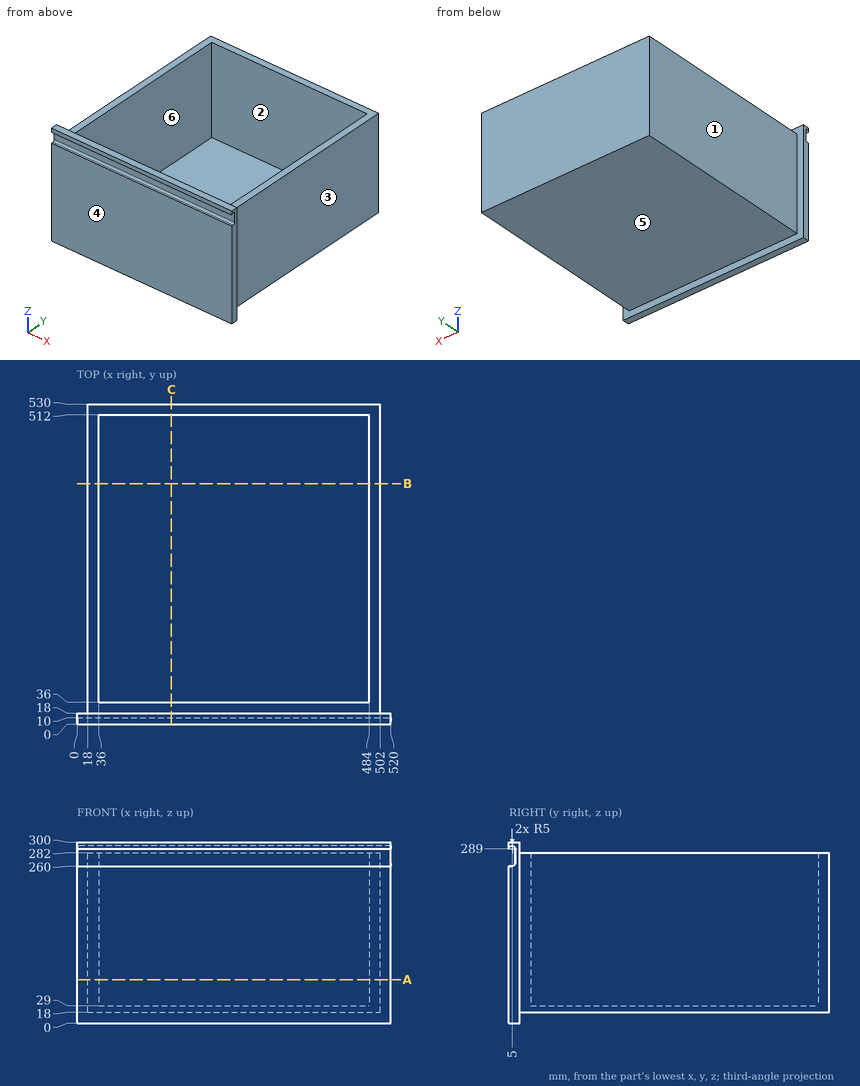
Could you check a few things on this drawing? It's one solid part, dimensions in mm from its lowest x, y, z. A direction names the side the tool comes from. Coordinates: 2 decimals unless noted, no trailing zeros. Write each loop counter-clockwise with the first axis right and the second up, starting at its lowest first coordinate (ties: lowest second). Pieces come first, ordered by that corner, then holes.
Q1. Imagine slicing it at A-A, the plane z = 72. List the corners of the cut face in (x, y) for me.
Results found:
outline: (0, 0) - (520, 0) - (520, 18) - (502, 18) - (502, 530) - (18, 530) - (18, 18) - (0, 18) - close; hole (36, 36) - (484, 36) - (484, 512) - (36, 512) - close
Q2. Which directions (+Z, -Z, +X, -X, +Y, -Y) give clear straight access to the entire face, cutting with the end or side of a thin tool? Please do the marked faces 1, 2 and 3.
Results found:
face 1: +Z, -Z, -X, +Y
face 2: +Z
face 3: +Z, -Z, +X, +Y
Q3. Please list where these lines run through material, in increasing order: L1, parallel to X at y = 79, z = 33.5; L2, parallel to Y at x = 245, z = 187; L3, parallel to Z at x = 227, y = 449.
Results found:
L1: x = 18 to 36, 484 to 502
L2: y = 0 to 36, 512 to 530
L3: z = 18 to 29
Q4. Imagine slicing it at C-C, the plane x = 156.5. List the corners of the cut face in (y, z) for me, plus the area to 3 significant figures.
Results found:
outline: (0, 0) - (18, 0) - (18, 18) - (530, 18) - (530, 282) - (512, 282) - (512, 29) - (36, 29) - (36, 282) - (18, 282) - (18, 300) - (0, 300) - (0, 289) arc R5 cw to (10, 289) - (10, 265) arc R5 cw to (5, 260) - (0, 260) - close
area: 19,800 mm2
Q5. Imagine slicing it at B-B, the plane y = 398. List the corners of the cut face in (x, z) for me.
Results found:
outline: (18, 18) - (502, 18) - (502, 282) - (484, 282) - (484, 29) - (36, 29) - (36, 282) - (18, 282) - close
Q6. If we mould it in two halves opening along Y, with no side actions, what happens to the marked faces 4, 5 and 6? For each: +Y half, -Y half, draft (parallel to the pull), parting line (faces both ways), or undercut.
Results found:
face 4: -Y half
face 5: draft
face 6: undercut
Q7. For P1, Ø8, axis at x = 376, y = 474.5, coming from the -Z side; P2, Ø6, axis at x = 137, y = 164, coming from the +Z side; P3, Ø1, axis at y = 100, z = 151.5, coming from the -X side, each with a flat end and sliding along its axis, tell me the tip position at first contact or that it passes through.
Results found:
P1: stops at z = 18
P2: stops at z = 29
P3: stops at x = 18
